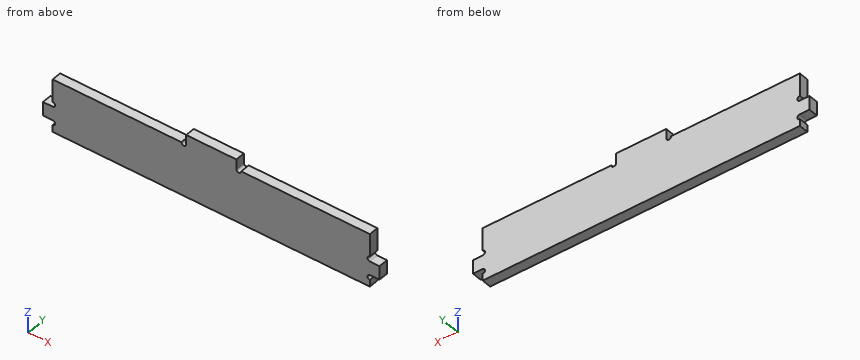
Autodesk Inventor part; units mm, degrees
ref_plane "YZ Plane" through (0, 0, 0) normal (1, 0, 0) x (0, 1, 0)
ref_plane "XZ Plane" through (0, 0, 0) normal (0, 1, 0) x (-1, 0, 0)
ref_plane "XY Plane" through (0, 0, 0) normal (0, 0, 1) x (1, 0, 0)
sketch "Sketch1" plane through (0, 0, 0) normal (0, 1, 0) x (-1, 0, 0)
  arc A0 (54.4292, -38.5976) -> (54.4292, -42.0976) centre (54.4292, -40.3476) ccw
  arc A1 (54.4292, -25.0976) -> (54.4292, -28.5976) centre (54.4292, -26.8476) ccw
  line L0 (61.4292, -38.5976) -> (61.4292, -28.5976)
  line L1 (-79.1541, -1.5976) -> (-42.6541, -1.5976)
  line L2 (-79.1541, -8.5976) -> (-79.1541, -1.5976)
  line L3 (-42.6541, -8.5976) -> (-42.6541, -1.5976)
  line L4 (61.4292, -28.5976) -> (54.4292, -28.5976)
  line L5 (61.4292, -38.5976) -> (54.4292, -38.5976)
  line L6 (54.4292, -25.0976) -> (54.4292, -8.5976)
  line L7 (54.4292, -42.0976) -> (54.4292, -47.0976)
  line L8 (-60.9041, -44.0976) -> (-60.9041, -33.5976)
  arc A2 (-176.2375, -42.0976) -> (-176.2375, -38.5976) centre (-176.2375, -40.3476) ccw
  arc A3 (-176.2375, -28.5976) -> (-176.2375, -25.0976) centre (-176.2375, -26.8476) ccw
  line L9 (-183.2375, -38.5976) -> (-183.2375, -28.5976)
  line L10 (-183.2375, -28.5976) -> (-176.2375, -28.5976)
  line L11 (-183.2375, -38.5976) -> (-176.2375, -38.5976)
  line L12 (-176.2375, -25.0976) -> (-176.2375, -8.5976)
  line L13 (-176.2375, -42.0976) -> (-176.2375, -47.0976)
  line L14 (54.4292, -47.0976) -> (-176.2375, -47.0976)
  arc A4 (-82.6541, -8.5976) -> (-79.1541, -8.5976) centre (-80.9041, -8.5976) ccw
  line L15 (-82.6541, -8.5976) -> (-176.2375, -8.5976)
  arc A5 (-42.6541, -8.5976) -> (-39.1541, -8.5976) centre (-40.9041, -8.5976) ccw
  line L16 (-39.1541, -8.5976) -> (54.4292, -8.5976)
  point P0 (0, 0)
  dimension "d2" = 3.5
  dimension "d5" = 3.5
  dimension "d9" = 7
  dimension "d11" = 10
  dimension "d27" = 36.5
  dimension "d32" = 5
  dimension "d33" = 230.6667
  dimension "d36" = 7
  dimension "d41" = 3.5
  dimension "d42" = 3.5
  dimension "d43" = 97.0833
extrude "Extrusion1" add sketch "Sketch1" along normal blind 7
properties part number "Level 1 Support Ends" material "Wood (Maple)"
CAD build for the part. Positions are in the model's coordinates, mm. Give positions to 0.01 mm unless a question says otherwise; leave off trailing zeros. Write each loop counter-clockwise with the first axis right and the second up, starting at its lowest first coordinate (ties: lowest second). Pieces come first, ordered by that corner, then holes. Notation, with made-up numbers: (38, 35.5) - (92, 35.5) arc R16 ccw to (92, 59.5) - close; hole circle Ø5 at (81, -37). An arc over 180 degrees is marked (long way). Put each result on its own line as item: value.
(1) Wall check: L1, parallel to X at y = 5.5, z = -25; L2, parallel to Z at x = 136, y = 1.25; L3, parallel to X at y = 3, z = -5.5. Give the ranges that are in metal, low to high.
Working result:
L1: -54.43 to 176.24
L2: -47.1 to -8.6
L3: 42.65 to 79.15
(2) Saw through at C-C (x = 153). List the corners of the cut face in (y, z), then the cut area to 4 significant figures.
Working result:
outline: (0, -47.1) - (7, -47.1) - (7, -8.6) - (0, -8.6) - close
area: 269.5 mm^2
(3) Saw through at A-A (y = 5). List the corners of the cut face in (x, z).
Working result:
outline: (-61.43, -38.6) - (-54.43, -38.6) arc R1.75 cw to (-54.43, -42.1) - (-54.43, -47.1) - (176.24, -47.1) - (176.24, -42.1) arc R1.75 cw to (176.24, -38.6) - (183.24, -38.6) - (183.24, -28.6) - (176.24, -28.6) arc R1.75 cw to (176.24, -25.1) - (176.24, -8.6) - (82.65, -8.6) arc R1.75 cw to (79.15, -8.6) - (79.15, -1.6) - (42.65, -1.6) - (42.65, -8.6) arc R1.75 cw to (39.15, -8.6) - (-54.43, -8.6) - (-54.43, -25.1) arc R1.75 cw to (-54.43, -28.6) - (-61.43, -28.6) - close
(4) Saw through at B-B (z = -5.5). List the corners of the cut face in (x, y), then the cut area to 4 significant figures.
Working result:
outline: (42.65, 0) - (79.15, 0) - (79.15, 7) - (42.65, 7) - close
area: 255.5 mm^2
(5) Drop flat-ended pins along their axis: pin 1 Ø2 at (x, z) = (87.5, -10.5) entering from -Y; pin 2 Ø3.5 at (y, z) = (4, -6.5) entering from +X; pin 3 Ø2 at (x, y) = (179.5, 4) entering from -Z; pin 4 Ø2 at (y, z) = (3.5, -13) entering from +X. Give the stop position or say it passes through.
Working result:
pin 1: y = 0
pin 2: x = 79.15
pin 3: z = -38.6
pin 4: x = 176.24
